Part model, mm, in its own coordinate system. A direction names the side the tool comes from. Give positions to 0.01 mm unless a question says otherwise; leave off trailing zeros. Order: outer loops, then holes, each group sorted by start corner. A loop starts at its lowest first (then second) coordinate and runs counter-clockwise, first axis right, second up. Notation, with made-up numbers: M 17,22 L 71,22 A30 cw 71,50 Z; hole C 83,-9 d3. An arc over 180 degrees is marked long. Return JSON: item names as keys, results as strings.
Autodesk Inventor part; units mm, degrees
ref_plane "YZ Plane" through (0, 0, 0) normal (1, 0, 0) x (0, 1, 0)
ref_plane "XZ Plane" through (0, 0, 0) normal (0, 1, 0) x (-1, 0, 0)
ref_plane "XY Plane" through (0, 0, 0) normal (0, 0, 1) x (1, 0, 0)
sketch "Sketch1" plane through (0, 0, 0) normal (0, 0, 1) x (1, 0, 0)
  line L0 (-12.7, -12.7) -> (12.7, -12.7)
  line L1 (12.7, -12.7) -> (12.7, 12.7)
  line L2 (12.7, 12.7) -> (-12.7, 12.7)
  line L3 (-12.7, -12.7) -> (12.7, 12.7) construction
  line L4 (12.7, -12.7) -> (-12.7, 12.7) construction
  line L5 (-12.7, 10.414) -> (10.414, 10.414)
  line L6 (10.414, 10.414) -> (10.414, -10.414)
  line L7 (10.414, -10.414) -> (-12.7, -10.414)
  line L8 (-12.7, 10.414) -> (-12.7, 12.7)
  line L9 (-12.7, -10.414) -> (-12.7, -12.7)
  point P0 (0, 0)
  dimension "l1" = 25.4
  dimension "l2" = 25.4
  dimension "wt" = 2.286
extrude "Extrusion1" add sketch "Sketch1" against normal blind 508
sketch "Sketch2" plane through (-12.7, 12.7, 0) normal (0, 1, 0) x (1, 0, 0)
  line L0 (25.4, 0) -> (0, 0)
  line L1 (25.4, 0) -> (25.4, 508)
  line L2 (0, 508) -> (25.4, 508)
  line L3 (0, 0) -> (0, 508)
  point P0 (12.7, 0)
  point P1 (12.7, 12.7)
  dimension "d5" = 25.4
  dimension "d7" = 12.7
  dimension "d8" = 12.7
hole "Hole1" at (0, 12.7, -12.7) direction (0, -1, 0) diameter 4.0894 end through all
sketch "Sketch3" plane through (12.7, -12.7, 0) normal (1, 0, 0) x (0, 0, -1)
  line L0 (0, 0) -> (0, 25.4)
  line L1 (0, 0) -> (508, 0)
  line L2 (508, 25.4) -> (508, 0)
  line L3 (0, 25.4) -> (508, 25.4)
  point P0 (0, 12.7)
  point P1 (12.7, 12.7)
  dimension "bot_dist" = 12.7
  dimension "d17" = 25.4
  dimension "d18" = 12.7
hole "Hole2" at (12.7, 0, -12.7) direction (-1, 0, 0) diameter 4.0894 end through all
sketch "Sketch4" plane through (12.7, -12.7, 0) normal (1, 0, 0) x (0, 0, -1)
  line L0 (0, 0) -> (0, 25.4)
  line L1 (0, 25.4) -> (508, 25.4)
  line L2 (0, 0) -> (508, 0)
  point P0 (0, 12.7)
  point P1 (12.7, 12.7)
  point P2 (12.7, 12.7)
  dimension "d26" = 12.7
  dimension "d27" = 12.7
  dimension "d28" = 12.7
hole "Hole3" [suppressed]
pattern_linear "Rectangular Pattern1" count 21 spacing 25.4 along (0, 0, -1) of "Hole1"
pattern_linear "Rectangular Pattern2" count 21 spacing 25.4 along (0, 0, -1) of "Hole2"
pattern_linear "Rectangular Pattern3" [suppressed]
chamfer "Chamfer1" distance 3.175 angle 45 4 edges at (-12.7, 11.557, 0) (-12.7, -11.557, 0) (-12.7, 11.557, -508) (-12.7, -11.557, -508)
fillet "Fillet1" radius 4.572 4 edges at (12.7, 12.7, -254) (12.7, -12.7, -254) (10.414, -10.414, -254) (10.414, 10.414, -254)
properties part number "channel-1x1x1-0001" material "Aluminum 5052-H36"
Q1. 3-axis set-ups, long thin cutter, end or side, ignore diameter. For faces 4 (the flat face through (-3, -10.414, -250)), 5 (the flat face through (12.7, 0, -250)): which of +Z, -Z, +X, -X, +Y, -Y reach the whole face in a straight line?
Established:
{"face 4": "+Z, -Z, -X", "face 5": "+Z, -Z, +X, +Y, -Y"}
Q2. Pin check, flat tips, straight feed: pin 1 (5.5 mm diameter, centred on x = 0, z = -342.9, fed in from +Y); pin 2 (6 mm diameter, centred on y = 1.5, z = -323.5, fed in from -X). Stop position of each tip, or through.
Established:
{"pin 1": "stops at y = 12.7", "pin 2": "stops at x = 10.41"}
Q3. Two-plate mould, pull along Y, no slides. Class faces 1 (the flat face through (-4, 10.414, -250)), 2 (the flat face through (-2, -12.7, -250)), 3 (the flat face through (11, 0, 0)): +Y half, -Y half, draft (parallel to the pull), parting line (faces both ways), or undercut.
Established:
{"face 1": "undercut", "face 2": "-Y half", "face 3": "draft"}
Q4. Probe line 1 along Y through (x, z) = (-6.5, -192); line 2 along X through (y, z) = (-12.1, -342.9); line 3 along X through (y, z) = (-1, -237). List the from-to ranges inside material, lowest first.
Established:
{"line 1": "y = -12.7 to -10.41, 10.41 to 12.7", "line 2": "x = -12.7 to -2.04, 2.04 to 10.39", "line 3": "x = 10.41 to 12.7"}
Q5. Band-saw the part on A-A (z = -303.5). Give the cut face in (x, y), then the cut area to 3 significant figures.
Established:
{"outline": "M -12.7,-12.7 L 8.13,-12.7 A4.57 ccw 12.7,-8.13 L 12.7,8.13 A4.57 ccw 8.13,12.7 L -12.7,12.7 L -12.7,10.41 L 5.84,10.41 A4.57 cw 10.41,5.84 L 10.41,-5.84 A4.57 cw 5.84,-10.41 L -12.7,-10.41 Z", "area": "164 mm²"}
